```python
from build123d import *

# Parameters (mm, degrees)
F0_R     = 1.27
F1_DEPTH = 48.26
F2_R     = 0.889
F3_DEPTH = 98.552
F4_R     = 0.508
F5_DEPTH = 129.794


with BuildPart() as f1:
    # F0 (on Top) → F1 (new body)
    with BuildSketch(Plane.XY):
        Circle(F0_R)
    extrude(amount=F1_DEPTH)

    # F2 (on Top) → F3 (join)
    with BuildSketch(Plane.XY):
        Circle(F2_R)
    extrude(amount=F3_DEPTH)

    # F4 (on Top) → F5 (join)
    with BuildSketch(Plane.XY):
        Circle(F4_R)
    extrude(amount=F5_DEPTH)


solid = f1.part
```
CAD build for the part. Positions are in the model's coordinates, mm. Give positions to 0.01 mm unless a question says otherwise; leave off trailing zeros. Loops run counter-clockwise (first coordinate to the right, second up) from the corner with the lowest first, then second, coordinate; pieces in that order, holes last. Notation, with made-up numbers: (-37.75, -4.5) - (-6.75, -4.5) arc R20 cw to (-6.75, 0.5) - close; hole circle Ø7 at (58.25, 31). An arc over 180 degrees is marked (long way). Put each result on its own line as item: value.
Q1. Slice it at D-D (z = 13). Give the cut face in (x, y), plus the area to 3 significant figures.
Filled in:
outline: circle Ø2.54 at (0, 0)
area: 5.07 mm²
Q2. Slice it at C-C (z = 79.5). Give the cut face in (x, y), plus the area to 3 significant figures.
Filled in:
outline: circle Ø1.78 at (0, 0)
area: 2.48 mm²
Q3. Slice it at A-A (y = 0). Give the cut face in (x, z).
Filled in:
outline: (-1.27, 0) - (1.27, 0) - (1.27, 48.26) - (0.89, 48.26) - (0.89, 98.55) - (0.51, 98.55) - (0.51, 129.79) - (-0.51, 129.79) - (-0.51, 98.55) - (-0.89, 98.55) - (-0.89, 48.26) - (-1.27, 48.26) - close
Q4. Probe line 1 along X through (y, z) = (0.05, 24.5); line 2 along Y through (x, z) = (-0.15, 37); line 3 along X through (y, z) = (-0.1, 76). List the from-to ranges inside material, lowest first.
Filled in:
line 1: x = -1.27 to 1.27
line 2: y = -1.26 to 1.26
line 3: x = -0.88 to 0.88
